```python
from build123d import *

# Parameters (mm, degrees)
BOSS_EXTRUDE1_DEPTH      = 4
BOSS_EXTRUDE1_DEPTH_BACK = 4
SKETCH1_R                = 22.5
SKETCH1_R_2              = 7
SKETCH1_R_3              = 2
SKETCH1_R_4              = 2.5
SKETCH2_R                = 2
CUT_EXTRUDE1_DEPTH       = 4
CUT_EXTRUDE1_DEPTH_BACK  = 4


with BuildPart() as part:
    # Sketch1 → Boss-Extrude1 (new, two sides: drawn at the far end of the back side and taken through both)
    with BuildSketch(Plane(origin=(0, 0, 0), x_dir=(1, 0, 0), z_dir=(0, 1, 0)).offset(-BOSS_EXTRUDE1_DEPTH_BACK)):
        with Locations(Location((0, 0, 0), (0, 0, 270))):
            Circle(SKETCH1_R)
        with Locations(Location((0, 0, 0), (0, 0, 270))):
            Circle(SKETCH1_R_2, mode=Mode.SUBTRACT)
        with Locations(Location((0, 11.725, 0), (0, 0, 270))):
            Circle(SKETCH1_R_3, mode=Mode.SUBTRACT)
        with Locations(Location((11.725, 0, 0), (0, 0, 270))):
            Circle(SKETCH1_R_3, mode=Mode.SUBTRACT)
        with Locations(Location((0, -11.725, 0), (0, 0, 270))):
            Circle(SKETCH1_R_3, mode=Mode.SUBTRACT)
        with Locations(Location((-11.725, 0, 0), (0, 0, 270))):
            Circle(SKETCH1_R_3, mode=Mode.SUBTRACT)
        with Locations(Location((-12.374368671, 12.374368671, 0), (0, 0, 270))):
            Circle(SKETCH1_R_4, mode=Mode.SUBTRACT)
        with Locations(Location((12.374368671, -12.374368671, 0), (0, 0, 270))):
            Circle(SKETCH1_R_4, mode=Mode.SUBTRACT)
    extrude(amount=BOSS_EXTRUDE1_DEPTH + BOSS_EXTRUDE1_DEPTH_BACK)

    # Sketch2 → Cut-Revolve7 (revolve, cut)
    with BuildSketch(Plane.XY, mode=Mode.PRIVATE) as cut_revolve7_sk:
        with Locations((22.5, 0)):
            Circle(SKETCH2_R)
    revolve(cut_revolve7_sk.sketch.rotate(Axis((0, 0, 0), (0, 1, 0)), 270), axis=Axis((0, 0, 0), (0, 1, 0)), mode=Mode.SUBTRACT)

    # Sketch3 → Cut-Extrude1 (cut, two sides: drawn at the far end of the back side and taken through both)
    with BuildSketch(Plane(origin=(0, 0, 0), x_dir=(1, 0, 0), z_dir=(0, 1, 0)).offset(-CUT_EXTRUDE1_DEPTH_BACK)):
        Polygon((-18.384776311, 16.263455967), (-13.435028843, 11.313708499), (-11.313708499, 13.435028843), (-16.263455967, 18.384776311), align=None)
        Polygon((13.435028843, -11.313708499), (11.313708499, -13.435028843), (16.263455967, -18.384776311), (18.384776311, -16.263455967), align=None)
    extrude(amount=CUT_EXTRUDE1_DEPTH + CUT_EXTRUDE1_DEPTH_BACK, mode=Mode.SUBTRACT)


solid = part.part
```
Here's how the part is built. I have some questions about the finished solid (model axes, mm). A direction names the side the tool comes from. Coordinates: 2 decimals unless noted, no trailing zeros. Order: outer loops, then holes, each group sorted by start corner. A loop starts at its lowest first (then second) coordinate and runs counter-clockwise, first axis right, second up.
1) Imagine slicing it at B-B on z = 0. List the corners of the cut face in (x, y) for me (3 decimals).
2) I need wall thicknesses on line 1 (X direction, y = 3, z = 0) (3 decimals); line 2 (X direction, y = 0.25, z = 0) (3 decimals); line 3 (Z direction, x = -1.5, y = -0.5). Which ranges of each line are inside material? Lowest first, please.
3) Which directions (+Z, -Z, +X, -X, +Y, -Y) give clear straight access to the entire face, cutting with the end or side of a thin tool? Please do faces 5 (the face through (15.21, -0.06, 13.09)), 6 (the face through (-0.77, -0.06, -9.88)), 7 (the face through (-15.21, -0.06, -13.09)), 8 (the face through (5.3, -4, -5.3)), 9 (the face through (-13.29, -0.06, -15.41)).
4) Imagine slicing it at A-A on x = 0. List the corners of the cut face in (y, z) for me (3 decimals), and give its area (3 significant figures).
5) Will these pins go through, and if not, where does the flat tip stop? pin 1 (2 mm diameter, centred on x = 6.5, y = 2.5, fed in from +Z); pin 2 (4 mm diameter, centred on y = -2.5, z = -8, fed in from -X); pin 3 (18 mm diameter, centred on x = 0, z = 0, fed in from +Y); pin 4 (4 mm diameter, centred on x = -6.5, y = -3, fed in from +Z).
6) Imagine slicing it at D-D on z = 10.5. State how many separate pieces and enclosed holes the cut face has, and give its area (3 significant figures).
7) We'd pull the mould along X, two halves only. Please class faces 1 (the face through (-10.669, -0.056, -10.546)), 2 (the face through (16.24, -3.01, -15.57)), 3 (the face through (13.29, -0.06, 15.41)), 4 (the face through (-6.834, -0.056, -1.517)): +X half, -X half, draft (parallel to the pull), parting line (faces both ways), or undercut.
Response values:
1. outline: (-22.5, -4) - (-13.725, -4) - (-13.725, 4) - (-22.5, 4) - (-22.5, 2) arc R2 cw to (-22.5, -2) - close; (-9.725, -4) - (-7, -4) - (-7, 4) - (-9.725, 4) - close; (7, -4) - (9.725, -4) - (9.725, 4) - (7, 4) - close; (13.725, -4) - (22.5, -4) - (22.5, -2) arc R2 cw to (22.5, 2) - (22.5, 4) - (13.725, 4) - close
2. line 1: x = -22.5 to -13.725, -9.725 to -7, 7 to 9.725, 13.725 to 22.5
2. line 2: x = -20.516 to -13.725, -9.725 to -7, 7 to 9.725, 13.725 to 20.516
2. line 3: z = -20.51 to -13.05, -10.4 to -6.84, 6.84 to 10.4, 13.05 to 20.51
3. face 5: +Z, +Y, -Y
3. face 6: +Y, -Y
3. face 7: -Z, +Y, -Y
3. face 8: +Z, -Z, +X, -X, -Y
3. face 9: -X, +Y, -Y
4. outline: (-4, -22.5) - (-2, -22.5) arc R2 cw to (2, -22.5) - (4, -22.5) - (4, -13.725) - (-4, -13.725) - close; (-4, -9.725) - (4, -9.725) - (4, -7) - (-4, -7) - close; (-4, 7) - (4, 7) - (4, 9.725) - (-4, 9.725) - close; (-4, 13.725) - (4, 13.725) - (4, 22.5) - (2, 22.5) arc R2 cw to (-2, 22.5) - (-4, 22.5) - close
4. area: 171 mm2
5. pin 1: stops at z = 21.82
5. pin 2: stops at x = -21.69
5. pin 3: stops at y = 4
5. pin 4: stops at z = 22.05
6. separate pieces: 3
6. enclosed holes: 0
6. area: 252 mm2
7. face 1: undercut
7. face 2: parting line
7. face 3: +X half
7. face 4: undercut
